Geometry: final body of the model. Coordinates: model frame, mm. A direction names the side the tool comes from. Give positions to 0.01 mm unless a question says otherwise; leave off trailing zeros. Write each loop counter-clockwise with the first axis right and the second up, starting at its lowest first coordinate (ties: lowest second). Pieces come first, ordered by that corner, then holes.
from build123d import *

# Parameters (mm, degrees)
EXTRUDE_1_DEPTH = 22.5
SKETCH_2_R      = 18
EXTRUDE_2_DEPTH = 100
CHAMFER_1_SIZE  = 2


# Read off the part's stored shape, not the designer's step: 切除-旋转-薄壁1
with BuildPart() as part:
    # 草图1 → 拉伸1 (new body)
    with BuildSketch(Plane.XY):
        Polygon((31.754264805, 0), (15.877132403, 27.5), (-15.877132403, 27.5), (-31.754264805, 0), (-15.877132403, -27.5), (15.877132403, -27.5), align=None)
    extrude(amount=EXTRUDE_1_DEPTH)

    # 草图2 → 拉伸2 (add)
    with BuildSketch(Plane.XY.offset(22.5)):
        with Locations(Location((0, 0, 0), (0, 0, 180))):
            Circle(SKETCH_2_R)
    extrude(amount=EXTRUDE_2_DEPTH)

    # 切除-旋转-薄壁1 outline → 切除-旋转-薄壁1 (revolve, cut)
    with BuildSketch(Plane.XZ):
        Polygon((31.754264936, 4.000000075), (24.826061575, 0), (31.754264936, 0), align=None)
    revolve(axis=Axis((0, 0, 0), (0, 0, 1)), mode=Mode.SUBTRACT)

    # 倒角1
    chamfer_1_edges = [part.edges().sort_by_distance(p)[0] for p in [
        (18, 0, 122.5),
    ]]
    chamfer(chamfer_1_edges, length=CHAMFER_1_SIZE)


solid = part.part
Q1. Section A-A on x = 0. Output: boundary loops of the cut face in (y, z).
Filled sheet:
outline: (-27.5, 1.54) - (-24.83, 0) - (24.83, 0) - (27.5, 1.54) - (27.5, 22.5) - (18, 22.5) - (18, 120.5) - (16, 122.5) - (-16, 122.5) - (-18, 120.5) - (-18, 22.5) - (-27.5, 22.5) - close
Q2. Ray query, line 1 along Z through (x, y) = (-11.5, -17); line 2 along Y through (x, z) = (3, 109.5); line 3 along X through (y, z) = (15, 107). Return the intervals inside material, ascending.
Filled sheet:
line 1: z = 0 to 22.5
line 2: y = -17.75 to 17.75
line 3: x = -9.95 to 9.95
Q3. Pin query (flat end, axial travel): P1, Ø6, axis at x = 17, z = 38, coming from the -Y side; P2, Ø4, axis at x = -22, y = -0.5, coming from the +Z side; P3, Ø4, axis at x = 0, z = 63.5, coming from the +Y side. Return the tip coordinate at first contact, or that it passes through.
Filled sheet:
P1: stops at y = -11.31
P2: stops at z = 22.5
P3: stops at y = 18
Q4. Access query for faces 1 (the flat face through (0, 27.5, 12)), 2 (the flat face through (14, 13, 22.5)). Directions: +Z, -Z, +X, -X, +Y, -Y. A direction counts if a zero-diameter tool reaches every point of the face in a straight line with its end or side. Return the directions, or none.
Filled sheet:
face 1: +Z, -Z, +X, -X, +Y
face 2: +Z
Q5. Section C-C on z = 103. Output: boundary loops of the cut face in (x, y).
Filled sheet:
outline: circle Ø36 at (0, 0)
Q6. Section B-B on z = 16. Output: boundary loops of the cut face in (x, y), plus the area to 3 significant figures.
Filled sheet:
outline: (-31.75, 0) - (-15.88, -27.5) - (15.88, -27.5) - (31.75, 0) - (15.88, 27.5) - (-15.88, 27.5) - close
area: 2,620 mm2
